```python
from build123d import *

# Parameters (mm, degrees)
SKETCH_W        = 19
SKETCH_H        = 14
PAD_DEPTH       = 9
SKETCH001_R     = 5
POCKET_DEPTH    = 9
SKETCH002_W     = 2
SKETCH002_H     = 14
PAD001_DEPTH    = 12
POCKET001_DEPTH = 19.001
SKETCH004_R     = 4
PAD002_DEPTH    = 4
SKETCH005_R     = 4
PAD003_DEPTH    = 4
SKETCH006_R     = 1.75
POCKET002_DEPTH = 27.001
POCKET003_DEPTH = 11
SKETCH008_W     = 4
SKETCH008_H     = 3
PAD004_DEPTH    = 3


with BuildPart() as part:
    # Sketch → Pad (new body)
    with BuildSketch(Plane.YZ):
        Rectangle(SKETCH_W, SKETCH_H)
    extrude(amount=PAD_DEPTH)

    # Sketch001 (on Face6 of Pad) → Pocket (cut)
    with BuildSketch(Plane.YZ.offset(9)):
        Circle(SKETCH001_R)
    extrude(amount=-POCKET_DEPTH, mode=Mode.SUBTRACT)

    # Sketch002 (on Face4 of Pocket) → Pad001 (join)
    with BuildSketch(Plane(origin=(0, 0, 0), x_dir=(0, 1, 0), z_dir=(-1, 0, 0))):
        with Locations((-8.5, 0)):
            Rectangle(SKETCH002_W, SKETCH002_H)
        with Locations((8.5, 0)):
            Rectangle(SKETCH002_W, SKETCH002_H)
    extrude(amount=PAD001_DEPTH)

    # Sketch003 (on Face9 of Pad001) → Pocket001 (cut, through all)
    with BuildSketch(Plane(origin=(0, -9.5, 0), x_dir=(0, 0, -1), z_dir=(0, -1, 0))):
        Polygon((-4, -12), (-7, -12), (-7, 0), align=None)
        Polygon((7, 0), (4, -12), (7, -12), align=None)
    extrude(amount=-POCKET001_DEPTH, mode=Mode.SUBTRACT)

    # Sketch004 (on Face2 of Pocket001) → Pad002 (join)
    with BuildSketch(Plane(origin=(0, -9.5, 0), x_dir=(0, 0, -1), z_dir=(0, -1, 0))):
        with Locations((0, -4.5)):
            Circle(SKETCH004_R)
    extrude(amount=PAD002_DEPTH)

    # Sketch005 (on Face3 of Pad002) → Pad003 (join)
    with BuildSketch(Plane.ZX.offset(9.5)):
        with Locations((0, -4.5)):
            Circle(SKETCH005_R)
    extrude(amount=PAD003_DEPTH)

    # Sketch006 (on Face21 of Pad003) → Pocket002 (cut, through all)
    with BuildSketch(Plane.ZX.offset(13.5)):
        with Locations((0, -4.5)):
            Circle(SKETCH006_R)
    extrude(amount=-POCKET002_DEPTH, mode=Mode.SUBTRACT)

    # Sketch007 → Pocket003 (cut, symmetric)
    with BuildSketch(Plane.XZ):
        Polygon((-1.75, -1.587713), (-1.75, 1.587713), (-4.5, 3.175426), (-7.25, 1.587713), (-7.25, -1.587713), (-4.5, -3.175426), align=None)
    extrude(amount=POCKET003_DEPTH, both=True, mode=Mode.SUBTRACT)

    # Sketch008 (on DatumPlane) → Pad004 (join)
    with BuildSketch(Plane.YZ.offset(9)):
        Polygon((-4.5, 7), (-3.5, 12), (3.5, 12), (4.5, 7), (4.5, 6), (-4.5, 6), align=None)
        with Locations((0, 8.5)):
            Rectangle(SKETCH008_W, SKETCH008_H, mode=Mode.SUBTRACT)
        Polygon((4.5, -7), (3.5, -12), (-3.5, -12), (-4.5, -7), (-4.5, -6), (4.5, -6), align=None)
        with Locations((0, -8.5)):
            Rectangle(SKETCH008_W, SKETCH008_H, mode=Mode.SUBTRACT)
    extrude(amount=-PAD004_DEPTH)


solid = part.part
```
Design review of the part built by this model. Coordinates are the model's own, in mm. A direction names the side the tool comes from. Give positions to 0.01 mm unless a question says otherwise; leave off trailing zeros. Order: outer loops, then holes, each group sorted by start corner. A loop starts at its lowest first (then second) coordinate and runs counter-clockwise, first axis right, second up. Notation, with made-up numbers: (11.5, 76.25) -> (34.5, 76.25) arc R31 ccw to (34.5, 102.25) -> close; hole circle Ø1 at (27, 22.25). An arc over 180 degrees is marked (long way). Write item = value, one per line. Start each with the question number.
(1) We need section A-A on z = 8.25. Write out the cut boundary in (x, y).
(2) To check wall thickness, follow line 1 along Y through (x, z) = (-1.5, -4); line 2 along Z through (x, y) = (6.75, 0); line 3 along X through (y, z) = (-12.6, 0). State the ranges of each line that lie inside material, in increasing order.
(3) We need section D-D on z = 0. State how many separate pieces and enclosed holes the cut face has, plus the area to 3 significant figures.
(4) Mouldability with a two-part tool opening along Y and no side actions: class faces 1 (the face through (1, 9.5, 0)), 2 (the face through (6, 0, 11)), 3 (the face through (-5.8, -11, -1.4)) as +Y half, -Y half, draft (parallel to the pull), parting line (faces both ways), or undercut.
(5) We need section B-B on y = 0. Write out the cut boundary in (x, z), plus the area to 3 significant figures.
(6) For pin 1 (5.5 mm diameter, centred on y = 1, z = 9, fed in from -X); pin 2 (2.5 mm diameter, centred on x = 3.5, y = 2.5, fed in from +Z); pin 3 (1.5 mm diameter, centred on x = 7.5, z = 9, fed in from +Y), all flat-tipped, find the tip position at first contact; note any pin that passes through.
(7) For faces 4 (the face through (-8.405, -11.472, 0.867)), 5 (the face through (-7, -7.5, 2)), 6 (the face through (-3.106, 9.226, 2.37)), list the 3-axis set-ups (+Z, -Z, +X, -X, +Y, -Y) from which the entire face can be reached by the end or side of a thin tool; tool diameter is ignored.
(8) We need section C-C on x = 1. Write out the cut boundary in (y, z), plus the area to 3 significant figures.
Numbers:
q1.outline = (6, -4.25) -> (9, -4.25) -> (9, -2) -> (6, -2) -> close; (6, 2) -> (9, 2) -> (9, 4.25) -> (6, 4.25) -> close
q2.line_1 = -9.5 to -7.5, 7.5 to 9.5
q2.line_2 = -12 to -10, -7 to -5, 5 to 7, 10 to 12
q2.line_3 = -8.5 to -6.25, -2.75 to -0.5
q3.separate_pieces = 4
q3.enclosed_holes = 0
q3.area = 137 mm^2
q4.face_1 = +Y half
q4.face_2 = draft
q4.face_3 = undercut
q5.outline = (0, -7) -> (9, -7) -> (9, -5) -> (0, -5) -> close; (0, 5) -> (9, 5) -> (9, 7) -> (0, 7) -> close; (6, -12) -> (9, -12) -> (9, -10) -> (6, -10) -> close; (6, 10) -> (9, 10) -> (9, 12) -> (6, 12) -> close
q5.area = 48.0 mm^2
q6.pin_1 = 0
q6.pin_2 = 7
q6.pin_3 = 4.25
q7.face_4 = -Y
q7.face_5 = +Z, -Z, -X
q7.face_6 = none
q8.outline = (-9.5, -7) -> (9.5, -7) -> (9.5, 7) -> (-9.5, 7) -> close; hole circle Ø10 at (0, 0)
q8.area = 187 mm^2
